CAD build for the part. Positions are in the model's coordinates, mm. Round coordinates to 2 decimals unless told otherwise and drop trailing zeros. Order: outer loops, then holes, each group sorted by start corner. A loop starts at its lowest first (then second) coordinate and runs counter-clockwise, first axis right, second up. Notation, with made-up numbers: M 84,28.25 L 133,28.25 A25 cw 133,56.25 Z; hole C 80.25,58.25 d1. An arc over 180 degrees is marked long. Answer as a JSON object with one key per item and string values.
```python
from build123d import *

# Parameters (mm, degrees)
SKETCH1_W           = 100
SKETCH1_H           = 60
BOSS_EXTRUDE1_DEPTH = 3
SKETCH2_R           = 2
SKETCH2_R_2         = 1.5
CUT_EXTRUDE1_DEPTH  = 3
SKETCH3_W           = 23.5
SKETCH3_H           = 20.25
CUT_EXTRUDE2_DEPTH  = 10
CUT_EXTRUDE3_DEPTH  = 10
SKETCH5_W           = 28.25
SKETCH5_H           = 20.25
CUT_EXTRUDE4_DEPTH  = 10
SKETCH6_R           = 7
BOSS_EXTRUDE2_DEPTH = 3
SKETCH7_R           = 2
CUT_EXTRUDE6_DEPTH  = 3
SKETCH9_R           = 7
SKETCH9_R_2         = 2
BOSS_EXTRUDE3_DEPTH = 3
BOSS_EXTRUDE4_DEPTH = 3


with BuildPart() as part:
    # Sketch1 → Boss-Extrude1 (new body)
    with BuildSketch(Plane.XY):
        Rectangle(SKETCH1_W, SKETCH1_H)
    extrude(amount=BOSS_EXTRUDE1_DEPTH)

    # Sketch2 → Cut-Extrude1 (cut)
    with BuildSketch(Plane.XY.offset(3)):
        with Locations((-38, 0)):
            Circle(SKETCH2_R)
        with Locations((-18, 0)):
            Circle(SKETCH2_R)
        with Locations((12, 0)):
            Circle(SKETCH2_R)
        with Locations((-46, 26)):
            Circle(SKETCH2_R_2)
        with Locations((46, 26)):
            Circle(SKETCH2_R_2)
        with Locations((46, -26)):
            Circle(SKETCH2_R_2)
        with Locations((-46, -26)):
            Circle(SKETCH2_R_2)
    extrude(amount=-CUT_EXTRUDE1_DEPTH, mode=Mode.SUBTRACT)

    # Sketch3 → Cut-Extrude2 (cut)
    with BuildSketch(Plane.XY.offset(3)):
        with Locations((-3, 13.375)):
            Rectangle(SKETCH3_W, SKETCH3_H)
    cut_extrude2 = extrude(amount=-CUT_EXTRUDE2_DEPTH, mode=Mode.SUBTRACT)

    # Mirror1: Cut-Extrude2 across plane
    add(cut_extrude2.mirror(Plane.ZX), mode=Mode.SUBTRACT)

    # Sketch4 → Cut-Extrude3 (cut)
    with BuildSketch(Plane.XY.offset(3)):
        with BuildLine():
            Line((-21.25, 23.5), (-39.461651585, 23.5))
            ThreePointArc((-39.461651585, 23.5), (-41.050252532, 21.050252532), (-43.5, 19.461651585))
            Line((-43.5, 19.461651585), (-43.5, 4.330127019))
            ThreePointArc((-43.5, 4.330127019), (-37.356495502, 6.970358812), (-31.800201616, 3.25))
            Line((-31.800201616, 3.25), (-24.199798384, 3.25))
            ThreePointArc((-24.199798384, 3.25), (-22.949747468, 4.949747468), (-21.25, 6.199798384))
            Line((-21.25, 6.199798384), (-21.25, 23.5))
        make_face()
    cut_extrude3 = extrude(amount=-CUT_EXTRUDE3_DEPTH, mode=Mode.SUBTRACT)

    # Mirror2: Cut-Extrude3 across plane
    add(cut_extrude3.mirror(Plane.ZX), mode=Mode.SUBTRACT)

    # Sketch5 → Cut-Extrude4 (cut)
    with BuildSketch(Plane.XY.offset(3)):
        with Locations((29.375, 13.375)):
            Rectangle(SKETCH5_W, SKETCH5_H)
    cut_extrude4 = extrude(amount=-CUT_EXTRUDE4_DEPTH, mode=Mode.SUBTRACT)

    # Sketch6 → Boss-Extrude2 (add)
    with BuildSketch(Plane.XY.offset(3)):
        with Locations((-18, 0)):
            Circle(SKETCH6_R)
    extrude(amount=-BOSS_EXTRUDE2_DEPTH)

    # Sketch7 → Cut-Extrude6 (cut)
    with BuildSketch(Plane.XY.offset(3)):
        with Locations((-18, 0)):
            Circle(SKETCH7_R)
    extrude(amount=-CUT_EXTRUDE6_DEPTH, mode=Mode.SUBTRACT)

    # Mirror4: Cut-Extrude4 across plane
    add(cut_extrude4.mirror(Plane.ZX), mode=Mode.SUBTRACT)

    # Sketch9 → Boss-Extrude3 (add)
    with BuildSketch(Plane.XY.offset(3)):
        with Locations((12, 0)):
            Circle(SKETCH9_R)
        with Locations((12, 0)):
            Circle(SKETCH9_R_2, mode=Mode.SUBTRACT)
    extrude(amount=-BOSS_EXTRUDE3_DEPTH)

    # Sketch11 → Boss-Extrude4 (add)
    with BuildSketch(Plane.XY.offset(3)):
        with BuildLine():
            Line((43.5, 19.461651585), (43.5, 23.5))
            Line((43.5, 23.5), (39.461651585, 23.5))
            ThreePointArc((39.461651585, 23.5), (41.050252532, 21.050252532), (43.5, 19.461651585))
        make_face()
    boss_extrude4 = extrude(amount=-BOSS_EXTRUDE4_DEPTH)

    # Mirror5: Boss-Extrude4 across plane
    add(boss_extrude4.mirror(Plane.ZX))


solid = part.part
```
Item 1: Saw through at B-B on x = -18. List the corners of the cut face in (y, z).
Worked answers:
{"outline": "M -30,0 L -2,0 L -2,3 L -30,3 Z; M 2,0 L 30,0 L 30,3 L 2,3 Z"}
Item 2: Wall check: line 1 along Y through (x, z) = (-46, 1.4); line 2 along Y through (x, z) = (-28, 1.4); line 3 along Y through (x, z) = (-38, 1.15). Give the ranges that are in metal, low to high. Write a range as [from, to].
Worked answers:
{"line 1": "y = [-30, -27.5], [-24.5, 24.5], [27.5, 30]", "line 2": "y = [-30, -23.5], [-3.25, 3.25], [23.5, 30]", "line 3": "y = [-30, -23.5], [-7, -2], [2, 7], [23.5, 30]"}
Item 3: Drop a flat-ended pin along its axis: pin 1 Ø6.5 at (x, y) = (-38, 0) entering from +Z. Give the stop position or say it passes through.
Worked answers:
{"pin 1": "stops at z = 3"}
Item 4: Saw through at C-C on y = 0. List the corners of the cut face in (x, z), and give its area (3 significant figures).
Worked answers:
{"outline": "M -50,0 L -40,0 L -40,3 L -50,3 Z; M -36,0 L -20,0 L -20,3 L -36,3 Z; M -16,0 L 10,0 L 10,3 L -16,3 Z; M 14,0 L 50,0 L 50,3 L 14,3 Z", "area": "264 mm2"}
Item 5: Two-plate mould, pull along X, no slides. Class faces 1 (the cylindrical face through (-23, 4.9, 1.5)), 2 (the flat face through (-1, 0, 0)), 3 (the flat face through (15.25, -15, 2)): released by +X, released by -X, zero draft, split by the parting line, or undercut.
Worked answers:
{"face 1": "undercut", "face 2": "zero draft", "face 3": "undercut"}
Item 6: Saw through at A-A on x = -46. List the corners of the cut face in (y, z), and give its area (3 significant figures).
Worked answers:
{"outline": "M -30,0 L -27.5,0 L -27.5,3 L -30,3 Z; M -24.5,0 L 24.5,0 L 24.5,3 L -24.5,3 Z; M 27.5,0 L 30,0 L 30,3 L 27.5,3 Z", "area": "162 mm2"}
Item 7: Saw through at D-D on y = 26. List the corners of the cut face in (x, z).
Worked answers:
{"outline": "M -50,0 L -47.5,0 L -47.5,3 L -50,3 Z; M -44.5,0 L 44.5,0 L 44.5,3 L -44.5,3 Z; M 47.5,0 L 50,0 L 50,3 L 47.5,3 Z"}
